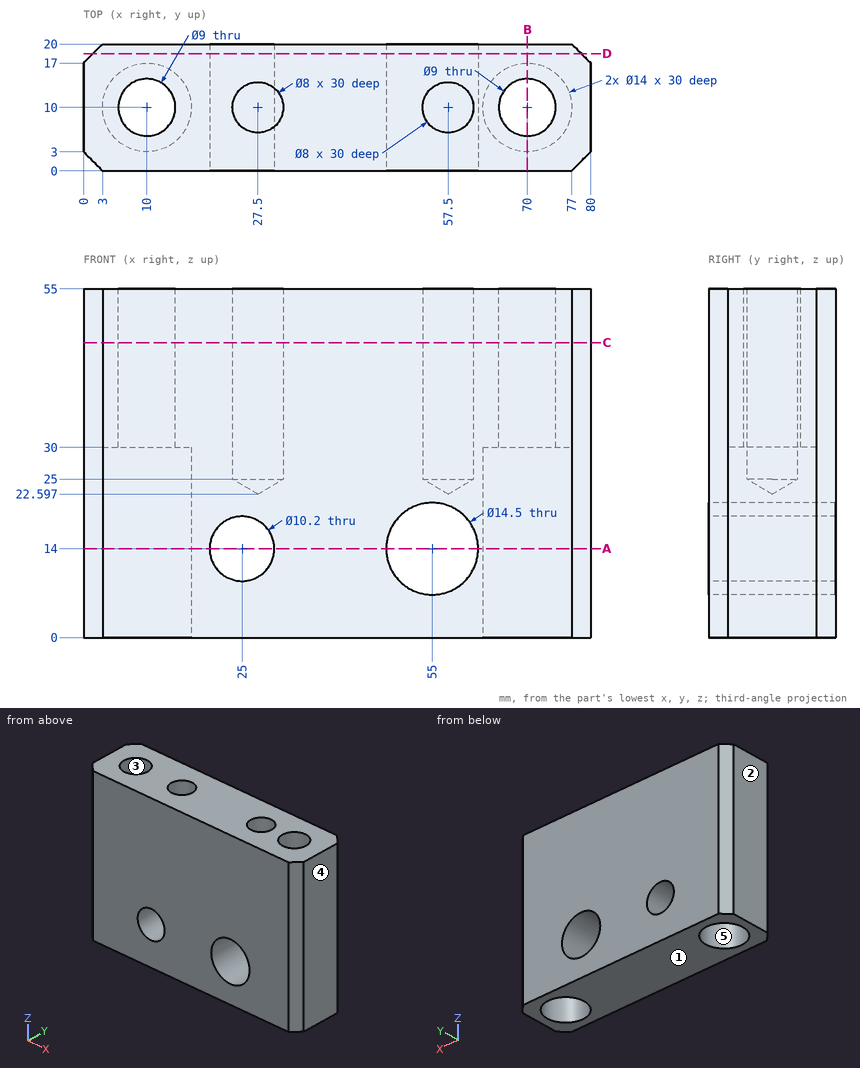
The figure shows three views and two pictorial views of one solid part (mm, origin at its lowest corner). Answer the questions. A direction names the side the tool comes from. Round coordinates to 2 decimals unless told otherwise and drop trailing zeros. Write each loop counter-clockwise with the first axis right and the second up, starting at its lowest first coordinate (ties: lowest second). Pieces come first, ordered by that corner, then holes. Notation, with made-up numbers: (39.25, -20) - (92.25, -20) arc R31 cw to (92.25, 14) - close; hole circle Ø8 at (86, 48). An arc over 180 degrees is marked (long way). One line per question, with ' | ' between items. Start each with the question number.
1. Section B-B (x = 70) is taken. Determine the outline of the cut face in (y, z).
2. Section C-C (z = 46.5) is taken. Determine the outline of the cut face in (x, y), and give its area (3 significant figures).
3. Section A-A (z = 14) is taken. Determine the outline of the cut face in (x, y), and give its area (3 significant figures).
4. Each of these flat-tipped pins is pushed along its axis until it touches: pin 1 (8.5 mm diameter, centred on x = 55, z = 14, fed in from +Y); pin 2 (6.5 mm diameter, centred on x = 27.5, y = 10, fed in from +Z). Where does it stop, or does it pass through?
5. For the marked faces 4 and 5, determine the directions among +Z, -Z, +X, -X, +Y, -Y from which every point of the face is accessible in a straight line to the end or side of a thin tool.
6. For a pull along X with two mould halves and no side action, classify the marked faces 1, 2 and 3 as +X half, -X half, draft (parallel to the pull), parting line (faces both ways), or undercut.
7. Section D-D (y = 18.5) is taken. Determine the outline of the cut face in (x, z).
8. Find the intervals of material crossed by probe 1 along X at (y, z) = (9.5, 3.5); probe 2 along X at (y, z) = (11.5, 32.5); probe 3 along Z at (x, y) = (69, 4), in increasing order. Write a range as [from, to].
Filled in:
1) outline: (0, 0) - (3, 0) - (3, 30) - (5.5, 30) - (5.5, 55) - (0, 55) - close; (14.5, 30) - (17, 30) - (17, 0) - (20, 0) - (20, 55) - (14.5, 55) - close
2) outline: (0, 3) - (3, 0) - (77, 0) - (80, 3) - (80, 17) - (77, 20) - (3, 20) - (0, 17) - close; hole circle Ø9 at (10, 10); hole circle Ø8 at (27.5, 10); hole circle Ø8 at (57.5, 10); hole circle Ø9 at (70, 10) | area: 1,350 mm²
3) outline: (0, 3) - (3, 0) - (19.9, 0) - (19.9, 20) - (3, 20) - (0, 17) - close; (30.1, 0) - (47.75, 0) - (47.75, 20) - (30.1, 20) - close; (62.25, 0) - (77, 0) - (80, 3) - (80, 17) - (77, 20) - (62.25, 20) - close; hole circle Ø14 at (10, 10); hole circle Ø14 at (70, 10) | area: 780 mm²
4) pin 1: through | pin 2: z = 24.55
5) face 4: +Z, -Z, +X, +Y, -Y | face 5: -Z
6) face 1: draft | face 2: -X half | face 3: undercut
7) outline: (1.5, 0) - (78.5, 0) - (78.5, 55) - (1.5, 55) - close; hole circle Ø10.2 at (25, 14); hole circle Ø14.5 at (55, 14)
8) probe 1: [0, 3.02], [16.98, 63.02], [76.98, 80] | probe 2: [0, 5.76], [14.24, 23.79], [31.21, 53.79], [61.21, 65.76], [74.24, 80] | probe 3: [30, 55]
